Design review of the part built by this model. Coordinates are the model's own, in mm. A direction names the side the tool comes from. Round coordinates to 2 decimals unless told otherwise and drop trailing zeros. Loops run counter-clockwise (first coordinate to the right, second up) from the corner with the lowest first, then second, coordinate; pieces in that order, holes last. Notation, with made-up numbers: M 76,11.5 L 93,11.5 A19 ccw 93,32.5 Z; hole C 45,66.25 d11. An arc over 180 degrees is marked long. Use a Markdown table: item, result.
Autodesk Inventor part; units mm, degrees
ref_plane "YZ Plane" through (0, 0, 0) normal (1, 0, 0) x (0, 1, 0)
ref_plane "XZ Plane" through (0, 0, 0) normal (0, 1, 0) x (-1, 0, 0)
ref_plane "XY Plane" through (0, 0, 0) normal (0, 0, 1) x (1, 0, 0)
sketch "Sketch3" plane through (0, 0, 0) normal (0, 1, 0) x (-1, 0, 0)
  line L0 (-57.5, 0) -> (57.5, 0)
  line L1 (62.5, -5) -> (62.5, -60)
  line L2 (-62.5, -45) -> (-62.5, -5)
  arc A0 (-57.5, 0) -> (-62.5, -5) centre (-57.5, -5) ccw
  arc A1 (62.5, -5) -> (57.5, 0) centre (57.5, -5) ccw
  line L3 (59.5, -60) -> (59.5, -5)
  arc A2 (59.5, -5) -> (57.5, -3) centre (57.5, -5) ccw
  line L4 (57.5, -3) -> (-57.5, -3)
  arc A3 (-57.5, -3) -> (-59.5, -5) centre (-57.5, -5) ccw
  line L5 (-59.5, -5) -> (-59.5, -45)
  line L6 (-62.5, -45) -> (-59.5, -45)
  line L7 (59.5, -60) -> (62.5, -60)
  point P0 (0, 0)
  point P1 (0, 0)
  dimension "d8" = 5
  dimension "d9" = 125
  dimension "d11" = 3
  dimension "d12" = 40
  dimension "d22" = 55
extrude "Extrusion3" add sketch "Sketch3" along normal blind 55
sketch "Sketch4" plane through (-57.5, 0, 0) normal (0, 0, 1) x (1, 0, 0)
  line L0 (0, 0) -> (115, 0)
  circle A0 centre (47.8, 28) radius 25
  line L1 (120, 0) -> (120, 55)
  line L2 (-5, 0) -> (-5, 55)
  point P0 (57.5, 0)
  dimension "d15" = 50
  dimension "d17" = 28
  dimension "d21" = 52.8
extrude "Extrusion4" cut sketch "Sketch4" against normal blind 60
properties part number "Beta_V2_BendFront01" material "Aluminum 6061 Black Anodized"
1. Insertion check: pin 1 (12 mm diameter, centred on x = 28.5, y = 27.5, fed in from -Z); pin 2 (1.5 mm diameter, centred on x = 60.5, y = 29.5, fed in from -Z). Each pin has a flat end and moves straight along its axis. Give the tip position at first contact, or say it passes through.
Check values:
| item | result |
|---|---|
| pin 1 | stops at z = -3 |
| pin 2 | stops at z = -45 |
2. Take a section at A-A on y = 28. Give the boundary of the cut face in (x, z), and give its area (3 significant figures).
Check values:
| item | result |
|---|---|
| outline | M -62.5,-60 L -59.5,-60 L -59.5,-5 A2 cw -57.5,-3 L -34.7,-3 L -34.7,0 L -57.5,0 A5 ccw -62.5,-5 Z; M 15.3,-3 L 57.5,-3 A2 cw 59.5,-5 L 59.5,-45 L 62.5,-45 L 62.5,-5 A5 ccw 57.5,0 L 15.3,0 Z |
| area | 513 mm² |
3. Machinability: for faces 1 (the face through (61, 27, -45)), 2 (the face through (59.5, 27, -25)), 3 (the face through (-61, 27, -60)), which of the approach directions +Z, -Z, +X, -X, +Y, -Y give a long, thin tool a straight path to every point of the face, cutting with its end or side? Answer none if there is none.
Check values:
| item | result |
|---|---|
| face 1 | -Z, +X, +Y, -Y |
| face 2 | -Z, +Y, -Y |
| face 3 | -Z, +X, -X, +Y, -Y |
4. Take a section at D-D on x = -52. Give the boundary of the cut face in (y, z), and give its area (3 significant figures).
Check values:
| item | result |
|---|---|
| outline | M 0,-3 L 55,-3 L 55,0 L 0,0 Z |
| area | 165 mm² |
5. Wall thickness on line 1 along Y through (x, z) = (-9, -2); line 2 along X through (y, z) = (42, -11); line 3 along Z through (x, y) = (-37, 27): over which ranges is each line inside the solid? List them lowest first. Write a range as from..to.
Check values:
| item | result |
|---|---|
| line 1 | y = 0..3.01, 52.99..55 |
| line 2 | x = -62.5..-59.5, 59.5..62.5 |
| line 3 | z = -3..0 |
6. Take a section at C-C on x = -9.7. Give the boundary of the cut face in (y, z).
Check values:
| item | result |
|---|---|
| outline | M 0,-3 L 3,-3 L 3,0 L 0,0 Z; M 53,-3 L 55,-3 L 55,0 L 53,0 Z |
7. Take a section at B-B on z = -14.5. Give the boundary of the cut face in (x, y).
Check values:
| item | result |
|---|---|
| outline | M -62.5,0 L -59.5,0 L -59.5,55 L -62.5,55 Z; M 59.5,0 L 62.5,0 L 62.5,55 L 59.5,55 Z |
